Geometry check sheet. Reference: the model listing, model coordinates, mm. A direction names the side the tool comes from. Round coordinates to 2 decimals unless told otherwise and drop trailing zeros. Write each loop counter-clockwise with the first axis right and the second up, starting at its lowest first coordinate (ties: lowest second). Pieces come first, ordered by that corner, then holes. Notation, with made-up numbers: M -16,44.5 L 21,44.5 A29 cw 21,70.5 Z; hole C 86.5,10.5 d5. An arc over 180 degrees is marked long. Answer in a Markdown table with one row per item. Add a question column.
from build123d import *

# Parameters (mm, degrees)
CROQUIS1_R              = 2.5
SALIENTE_EXTRUIR1_DEPTH = 85
CROQUIS2_R              = 1
CORTAR_EXTRUIR1_DEPTH   = 86
REDONDEO1_R             = 0.25
ENL_V_MAT_EXTRU_1_DEPTH = 25


with BuildPart() as part:
    # Croquis1 → Saliente-Extruir1 (new body)
    with BuildSketch(Plane.XY):
        Circle(CROQUIS1_R)
    extrude(amount=SALIENTE_EXTRUIR1_DEPTH)

    # Croquis2 → Cortar-Extruir1 (cut, through all)
    with BuildSketch(Plane.XY.offset(85)):
        Circle(CROQUIS2_R)
    extrude(amount=-CORTAR_EXTRUIR1_DEPTH, mode=Mode.SUBTRACT)

    # Redondeo1
    redondeo1_edges = [part.edges().sort_by_distance(p)[0] for p in [
        (-2.5, 0, 0),
        (-2.5, 0, 85),
        (-1, 0, 85),
    ]]
    fillet(redondeo1_edges, radius=REDONDEO1_R)

    # Esquisse1 → Enlèv. mat.-Extru.1 (cut)
    with BuildSketch(Plane.XY.offset(85)):
        with BuildLine():
            Line((-2.141675568, 1.289661103), (1.246569633, 2.167040413))
            ThreePointArc((1.246569633, 2.167040413), (-0.626699507, 2.420175144), (-2.141675568, 1.289661103))
        make_face()
    extrude(amount=-ENL_V_MAT_EXTRU_1_DEPTH, mode=Mode.SUBTRACT)


solid = part.part
Item 1: Access from +Z, -Z, +X, -X, +Y, -Y to the whole of each face (thin tool, end or side, straight path). Record for faces 1 (the flat face through (-0.471, 1.722, 72.675)), 2 (the flat face through (1, -1, 85)).
Item 2: Section check C-C, the plane x = 0. Record the boundary of the cut face in (y, z), and give its area (3 significant figures).
Item 3: Scan lines: probe 1 along Y at (x, z) = (0, 36); probe 2 along X at (y, z) = (0.45, 10.5); probe 3 along X at (y, z) = (-0.5, 59). Record each from-to range of solid material in increasing order. Write a range as from..to.
Item 4: Section check D-D, the plane z = 61. Record the boundary of the cut face in (x, y).
Item 5: Section check A-A, the plane y = 0. Record the boundary of the cut face in (x, z), and give its area (3 significant figures).
Item 6: Section check B-B, the plane z = 25.5. Record the boundary of the cut face in (x, y).
Item 7: Gauge pin test, flat ends, axial feed: pin 1 Ø1 at (x, y) = (0.5, 1) entering from -Z; pin 2 Ø2 at (y, z) = (-2, 33.5) entering from -X; pin 3 Ø1.6 at (x, y) = (0, 0) entering from +Z; pin 4 Ø1.5 at (x, z) = (2, 11.5) entering from +Y. Record the tip position at first contact, or that the pin passes through.
Result sheet:
| question | item | result |
|---|---|---|
| 1 | face 1 | +Z, -X, +Y |
| 1 | face 2 | +Z, +X, -X, +Y, -Y |
| 2 | outline | M -2.5,0.25 A0.25 ccw -2.25,0 L -1,0 L -1,84.75 A0.25 ccw -1.25,85 L -2.25,85 A0.25 ccw -2.5,84.75 Z; M 1,0 L 2.25,0 A0.25 ccw 2.5,0.25 L 2.5,60 L 1.84,60 L 1.84,85 L 1.25,85 A0.25 ccw 1,84.75 Z |
| 2 | area | 239 mm^2 |
| 3 | probe 1 | y = -2.5..-1, 1..2.5 |
| 3 | probe 2 | x = -2.46..-0.89, 0.89..2.46 |
| 3 | probe 3 | x = -2.45..-0.87, 0.87..2.45 |
| 4 | outline | M -2.14,1.29 A2.5 ccw long 1.25,2.17 Z; hole C 0,0 d2 |
| 5 | outline | M -2.5,0.25 A0.25 ccw -2.25,0 L -1,0 L -1,84.75 A0.25 ccw -1.25,85 L -2.25,85 A0.25 ccw -2.5,84.75 Z; M 1,0 L 2.25,0 A0.25 ccw 2.5,0.25 L 2.5,84.75 A0.25 ccw 2.25,85 L 1.25,85 A0.25 ccw 1,84.75 Z |
| 5 | area | 255 mm^2 |
| 6 | outline | C 0,0 d5; hole C 0,0 d2 |
| 7 | pin 1 | stops at z = 0 |
| 7 | pin 2 | stops at x = -2.29 |
| 7 | pin 3 | passes through |
| 7 | pin 4 | stops at y = 2.17 |
